from build123d import *

# Parameters (mm, degrees)
F0_W     = 30
F0_H     = 10
F1_DEPTH = 3
F2_W     = 34
F2_H     = 10
F3_DEPTH = 5
F4_W     = 30
F4_H     = 10
F5_DEPTH = 2
F6_W     = 30
F6_H     = 10
F7_DEPTH = 1


with BuildPart() as f1:
    # F0 (on Top) → F1 (new body)
    with BuildSketch(Plane.XY):
        Rectangle(F0_W, F0_H)
    extrude(amount=F1_DEPTH)

    # F2 (on face) → F3 (join)
    with BuildSketch(Plane.XY.offset(3)):
        Rectangle(F2_W, F2_H)
    extrude(amount=F3_DEPTH)

    # F4 (on face) → F5 (join)
    with BuildSketch(Plane.XY.offset(8)):
        Rectangle(F4_W, F4_H)
    extrude(amount=F5_DEPTH)

    # F6 (on face) → F7 (join)
    with BuildSketch(Plane.XY.offset(10)):
        Rectangle(F6_W, F6_H)
    extrude(amount=F7_DEPTH)


solid = f1.part
Can you work these out from the model? Positions are in its coordinate system, mm. A direction names the side the tool comes from. Give positions to 0.01 mm unless a question says otherwise; leave off trailing zeros. Write each loop counter-clockwise with the first axis right and the second up, starting at its lowest first coordinate (ties: lowest second). Pieces come first, ordered by that corner, then holes. Notation, with made-up numbers: (67, 54) -> (82, 54) arc R18 ccw to (82, 88) -> close; hole circle Ø10 at (26, 53). An arc over 180 degrees is marked (long way). Answer as a JSON object with one key per item and string values. Group by question number.
Item 1: For faces 4 (the face through (15, 0, 9)), 5 (the face through (-15, 0, 9)), 6 (the face through (-16, 0, 3)), 7 (the face through (16, 0, 3)), 8 (the face through (17, 0, 5)), which set-ups out of +Z, -Z, +X, -X, +Y, -Y let a thin tool reach every point of the face, with its end or its side?
Item 2: Suppose I cut it at A-A (y = 1). Please give me the cut outline in (x, z), plus the area to 3 significant figures.
Item 3: I'm going to push flat-ended pins straight in: P1, Ø1, axis at y = 1, z = 2, coming from the +X side; P2, Ø3.5, axis at y = 1.5, z = 1, coming from the -X side. Where does each tip first touch, or does it pass through?
Item 4: Suppose I cut it at B-B (z = 1). Please give me the cut outline in (x, y).
Item 5: We'd pull the mould along Y, two halves only. Please class faces 1 (the face through (0, 5, 5)), 2 (the face through (0, 0, 0)), 3 (the face through (0, -5, 5)): +Y half, -Y half, draft (parallel to the pull), parting line (faces both ways), or undercut.
Item 6: Please list where these lines run through material, in increasing order: line 1 (X direction, y = 3.5, z = 8.25); line 2 (Z direction, x = 15.5, y = 2.75). Write a range as [from, to].
Findings:
{
 "1": {"face 4": "+Z, +X, +Y, -Y", "face 5": "+Z, -X, +Y, -Y", "face 6": "-Z, -X, +Y, -Y", "face 7": "-Z, +X, +Y, -Y", "face 8": "+Z, -Z, +X, +Y, -Y"},
 "2": {"outline": "(-17, 3) -> (-15, 3) -> (-15, 0) -> (15, 0) -> (15, 3) -> (17, 3) -> (17, 8) -> (15, 8) -> (15, 11) -> (-15, 11) -> (-15, 8) -> (-17, 8) -> close", "area": "350 mm²"},
 "3": {"P1": "stops at x = 15", "P2": "stops at x = -15"},
 "4": {"outline": "(-15, -5) -> (15, -5) -> (15, 5) -> (-15, 5) -> close"},
 "5": {"face 1": "+Y half", "face 2": "draft", "face 3": "-Y half"},
 "6": {"line 1": "x = [-15, 15]", "line 2": "z = [3, 8]"}
}
